Design review of the part built by this model. Coordinates are the model's own, in mm. Coordinates: 2 decimals unless noted, no trailing zeros. Write each loop counter-clockwise with the first axis right and the second up, starting at its lowest first coordinate (ties: lowest second). Pieces come first, ordered by that corner, then holes. Notation, with made-up numbers: (89.25, 81) -> (100.25, 81) arc R14 cw to (100.25, 108) -> close; hole circle Ø4 at (-6, 24.5). An arc over 180 degrees is marked (long way). Answer in a Markdown table with one row per item. Add a question column.
Item 1: Clearance check with flat-ended pins moving along their axes: P1, Ø4.5, axis at x = 13.51, z = 4.39, coming from the -Y side; P2, Ø1, axis at x = -4, y = 2.5, coming from the +Z side; P3, Ø2, axis at x = -8.5, y = 3, coming from the +Z side; P4, Ø1, axis at x = 2.5, y = 1, coming from the -Z side. State where each tip first meets the part, or that it passes through.
Item 2: Take a section at D-D, the plane z = 5. Write out the cut boundary in (x, y).
Item 3: To check wall thickness, follow line 1 (Z direction, x = 8, y = 3.2); line 2 (Z direction, x = -14, y = 2.1); line 3 (X direction, y = 1, z = -10.5). State the ranges of each line that lie inside material, in increasing order.
Item 4: Draft analysis for pull direction X (two halves, no side actions). For faces 1 (the face through (-0.785, 1.972, -18.383)), 2 (the face through (8.996, 1.972, -12.735)), 3 (the face through (3.8, 0, 8.4)), 4 (the face through (-13.08, 2.03, -3.92)), state which applies: released by +X, released by -X, zero draft, split by the parting line, or undercut.
Item 5: Take a section at A-A, the plane x = 0. Write out the cut boundary in (y, z), and give its area (3 significant figures).
Item 6: Take a section at B-B, the plane z = 0. Write out the cut boundary in (x, y), and give its area (3 significant figures).
Item 7: Take a section at C-C, the plane y = 1.95. Give the number of separate pieces and of enclosed holes in the cut face, and give its area (3 significant figures).
from build123d import *

# Parameters (mm, degrees)
F0_R     = 18.4
F0_R_2   = 1.4
F0_R_3   = 9
F1_DEPTH = 4
F2_R     = 1.85
F3_DEPTH = 25
F5_DEPTH = 25


with BuildPart() as f1:
    # F0 (on Front) → F1 (new body)
    with BuildSketch(Plane.XZ):
        Circle(F0_R)
        with Locations((-8.35, -11.4927890359)):
            Circle(F0_R_2, mode=Mode.SUBTRACT)
        with Locations((8.35, -11.4927890359)):
            Circle(F0_R_2, mode=Mode.SUBTRACT)
        with Locations((-13.5105838061, 4.3898547862)):
            Circle(F0_R_2, mode=Mode.SUBTRACT)
        Circle(F0_R_3, mode=Mode.SUBTRACT)
        with Locations((13.5105838061, 4.3898547862)):
            Circle(F0_R_2, mode=Mode.SUBTRACT)
        with Locations((0, 14.2058684995)):
            Circle(F0_R_2, mode=Mode.SUBTRACT)
    extrude(amount=-F1_DEPTH)

    # F2 (on face) → F3 (cut)
    with BuildSketch(Plane(origin=(0, 4, 0), x_dir=(-1, 0, 0), z_dir=(0, 1, 0))):
        with Locations((-14.9282032303, -4)):
            Circle(F2_R)
        with Locations((-10.9282032303, 10.9282032303)):
            Circle(F2_R)
        with Locations((14.9282032303, -4)):
            Circle(F2_R)
        with Locations((10.9282032303, 10.9282032303)):
            Circle(F2_R)
        with Locations((4, -14.9282032303)):
            Circle(F2_R)
        with Locations((-4, -14.9282032303)):
            Circle(F2_R)
    extrude(amount=-F3_DEPTH, mode=Mode.SUBTRACT)

    # F4 (on face) → F5 (cut)
    with BuildSketch(Plane.XZ):
        with BuildLine():
            ThreePointArc((1.6850467371, 18.3226804124), (0, 18.4), (-1.6850467371, 18.3226804124))
            ThreePointArc((-1.6850467371, 18.3226804124), (0, 17.4), (1.6850467371, 18.3226804124))
        make_face()
    extrude(amount=-F5_DEPTH, mode=Mode.SUBTRACT)


solid = f1.part
Answers:
| question | item | result |
|---|---|---|
| 1 | P1 | stops at y = 0 |
| 1 | P2 | stops at z = 18.06 |
| 1 | P3 | stops at z = 16.8 |
| 1 | P4 | stops at z = -18.29 |
| 2 | outline | (-17.71, 0) -> (-14.77, 0) -> (-14.77, 4) -> (-17.71, 4) -> close; (-12.25, 0) -> (-7.48, 0) -> (-7.48, 4) -> (-12.25, 4) -> close; (7.48, 0) -> (12.25, 0) -> (12.25, 4) -> (7.48, 4) -> close; (14.77, 0) -> (17.71, 0) -> (17.71, 4) -> (14.77, 4) -> close |
| 3 | line 1 | z = -16.57 to -12.85, -10.14 to -4.12, 4.12 to 16.57 |
| 3 | line 2 | z = -11.94 to -5.6, -2.4 to 3.08, 5.7 to 11.94 |
| 3 | line 3 | x = -15.11 to -9.34, -7.36 to 7.36, 9.34 to 15.11 |
| 4 | face 1 | split by the parting line |
| 4 | face 2 | undercut |
| 4 | face 3 | zero draft |
| 4 | face 4 | undercut |
| 5 | outline | (0, -18.4) -> (4, -18.4) -> (4, -9) -> (0, -9) -> close; (0, 9) -> (4, 9) -> (4, 12.81) -> (0, 12.81) -> close; (0, 15.61) -> (4, 15.61) -> (4, 17.4) -> (0, 17.4) -> close |
| 5 | area | 60.0 mm^2 |
| 6 | outline | (-18.4, 0) -> (-9, 0) -> (-9, 4) -> (-18.4, 4) -> close; (9, 0) -> (18.4, 0) -> (18.4, 4) -> (9, 4) -> close |
| 6 | area | 75.2 mm^2 |
| 7 | separate pieces | 1 |
| 7 | enclosed holes | 12 |
| 7 | area | 711 mm^2 |
